The listing builds one solid part. Answer for the finished solid, in the listing's coordinates (mm). Face numbers are marked on the shaded views. A direction names the side the tool comes from. Round coordinates to 2 decimals unless told otherwise and drop trailing zeros. Order: outer loops, then holes, each group sorted by start corner. A loop starts at its lowest first (then second) coordinate and runs counter-clockwise, first axis right, second up. Notation, with made-up numbers: (-21, 56.25) -> (1, 56.25) arc R9 ccw to (1, 73.25) -> close; hole circle Ø2 at (28, 35.5). An arc over 180 degrees is marked (long way). Return JSON: item names as keys, results as strings. Group by question number.
(1) Each of these flat-tipped pins is pushed along its axis until it touches: pin 1 (1 mm diameter, centred on x = 22.5, y = 32, fed in from +Z); pin 2 (6 mm diameter, centred on x = 8, y = 7.5, fed in from -Z); pin 3 (3.5 mm diameter, centred on x = 0, z = 5, fed in from -Y); pin 4 (3 mm diameter, centred on y = 41, z = 48.5, fed in from +X). Where does it stop, or does it pass through?
(2) Determine the mould class of the marked faces 4, 5 and 6 for opening direction Y: +Y half, -Y half, draft (parallel to the pull), parting line (faces both ways), or undercut.
(3) Consider line 1 (X direction, y = -7.5, z = 28); line 2 (Z direction, x = 0, y = 8.35); line 3 (Z direction, x = 0, y = -8.7). Determine where each line is inside the solid, lowest interval first. Write a range as [from, to].
(4) Which of the six approach directions +Z, -Z, +X, -X, +Y, -Y give full straight-line access (tool end or side, diameter ignored) to the marked faces 1, 2 and 3?
(5) The part is cut by section B-B (x = 0). Determine the outline of the cut face in (y, z), plus the area to 3 significant figures.
(6) The part is cut by section C-C (y = 0). Determine the outline of the cut face in (x, z), plus the area to 3 significant figures.
(7) The part is cut by section D-D (x = 15). Determine the outline of the cut face in (y, z).
Autodesk Inventor part; units mm, degrees
ref_plane "Plan de construction2" through (0, -8.75, 15.1554) normal (0, -0.5, 0.8660254) x (1, 0, 0)
ref_plane "Plan de construction4" through (0, -10, 10) normal (0, -0.7071068, 0.7071068) x (1, 0, 0)
ref_plane "Plan de construction7" through (0, 10, 30) normal (0, -0.5, 0.8660254) x (1, 0, 0)
sketch "Esquisse1" plane through (0, 0, 0) normal (0, 0, 1) x (1, 0, 0)
  circle A0 centre (0, 0) radius 8
  circle A1 centre (0, 0) radius 9
  dimension "d0" = 16
  dimension "d1" = 18
extrude "Extrusion1" add sketch "Esquisse1" along normal blind 10
sketch "Esquisse2" plane through (0, 0, 0) normal (1, 0, 0) x (0, 1, 0)
  line L0 (9, 10) -> (-9, 10)
  line L1 (0, 10) -> (0, 25)
  line L2 (9, 10) -> (-9, 10)
  line L3 (0, 10) -> (10, 10)
  line L4 (10, 10) -> (10, 30)
  line L5 (10, 30) -> (-10, 30)
  line L6 (-10, 30) -> (-10, 10)
  line L7 (-10, 10) -> (0, 10)
  point P0 (0, 0)
  dimension "d26" = 10
  dimension "d27" = 20
  dimension "d28" = 20
  dimension "d29" = 90
extrude "Extrusion2" add sketch "Esquisse2" along normal mid plane 20
fillet "Congé1" radius 2 1 edges at (-9, 0, 10)
sketch "Esquisse4" plane through (0, 0, 0) normal (0, 1, 0) x (-1, 0, 0)
  line L0 (9, 0) -> (-9, 0)
  line L1 (9, 0) -> (0, 0)
  line L2 (0, 0) -> (0, 5)
  line L3 (0, 0) -> (5, 0) construction
  dimension "d14" = 9
  dimension "d15" = 5
  dimension "d16" = 90
hole "Perçage1" at (0, 0, 5) direction (0, -1, 0) diameter 4 end through all both
ref_plane "Plan de construction2" through (0, -8.75, 15.1554) normal (0, -0.5, 0.8660254) x (1, 0, 0)
ref_plane "Plan de construction1" through (0, 0, 0) normal (0, -0.5, 0.8660254) x (1, 0, 0)
ref_plane "Plan de construction4" through (0, -10, 10) normal (0, -0.7071068, 0.7071068) x (1, 0, 0)
ref_plane "Plan de construction3" through (0, 0, 0) normal (0, -0.7071068, 0.7071068) x (1, 0, 0)
sketch "Esquisse6" plane through (0, -10, 10) normal (0, -0.7071068, 0.7071068) x (1, 0, 0)
  line L0 (-10, 28.2843) -> (-10, 14.1421)
  line L1 (10, 14.1421) -> (10, 0)
  line L2 (-10, 28.2843) -> (10, 28.2843)
  line L3 (10, 28.2843) -> (10, 0)
  line L4 (10, 0) -> (-10, 0)
  line L5 (-10, 0) -> (-10, 28.2843)
  line L6 (-10, 28.2843) -> (10, 28.2843)
  line L7 (10, 14.1421) -> (10, 28.2843)
  line L8 (4.5826, 14.1421) -> (10, 14.1421)
  line L9 (-10, 14.1421) -> (-4.5826, 14.1421)
  line L10 (-10, 28.2843) -> (-10, 14.1421)
  point P0 (0, 0)
extrude "Extrusion4" add sketch "Esquisse6" along normal blind 25
fillet "Congé4" radius 20 1 edges at (0, -27.6777, 27.6777)
ref_plane "Plan de construction5" through (0, 10, 30) normal (0, 0.8660254, 0.5) x (1, 0, 0)
ref_plane "Plan de construction7" through (0, 10, 30) normal (0, -0.5, 0.8660254) x (1, 0, 0)
ref_plane "Plan de construction6" through (0, 1.3397, 25) normal (0, 0.8660254, 0.5) x (1, 0, 0)
sketch "Esquisse18" plane through (0, 1.3397, 25) normal (0, 0.8660254, 0.5) x (1, 0, 0)
  line L0 (10, -0.0001) -> (-10, -0.0001)
  line L1 (-10, -0.0001) -> (-10, -24.1482)
  line L2 (10, -24.1482) -> (-10, -24.1482)
  line L3 (10, -0.0001) -> (10, -24.1482)
  line L4 (10, -0.0001) -> (-10, -0.0001)
  line L5 (-10, -0.0001) -> (-10, -24.1482)
  line L6 (10, -24.1482) -> (-10, -24.1482)
  line L7 (10, -0.0001) -> (10, -24.1482)
  point P0 (0, 20.9808)
extrude "Extrusion14" add sketch "Esquisse18" along normal blind 60
fillet "Congé6" radius 5 1 edges at (0, -10.7344, 45.913)
sketch "Esquisse19" plane through (10, 0, 0) normal (1, 0, 0) x (0, 0, -1)
  line L0 (-30, 10) -> (-55.0001, 53.3012)
  line L1 (-55.0001, 53.3012) -> (-65.4564, 47.2642)
  line L2 (-47.3761, -8.2002) -> (-75.913, 41.2272)
  line L3 (-65.4564, 47.2642) -> (-58.4714, 35.1659)
  circle A0 centre (-58.4714, 35.1659) radius 4.1
  point P0 (0, 0)
  dimension "d76" = 12.074
  dimension "d77" = 13.97
  dimension "d78" = 8.2
extrude "Extrusion15" add sketch "Esquisse19" along normal blind 20
sketch "Esquisse20" plane through (10, 0, 0) normal (1, 0, 0) x (0, 0, -1)
  circle A0 centre (-58.4714, 35.1659) radius 4.1
  circle A1 centre (-58.4714, 35.1659) radius 4.75
  point P0 (0, 0)
  dimension "d81" = 9.5
extrude "Extrusion16" add sketch "Esquisse20" along normal blind 2
fillet "Congé7" radius 5 2 edges at (0, 53.3012, 55.0001) (0, 41.2272, 75.913)
properties part number "bielle roue milieu autre côté"
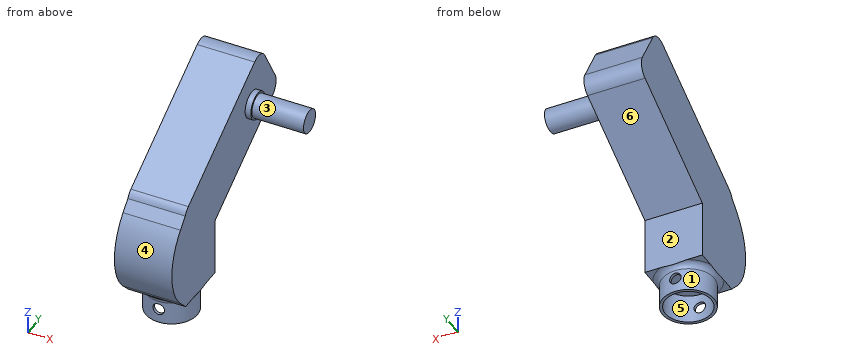
Answer below:
{
 "1": {"pin 1": "stops at z = 61.59", "pin 2": "stops at z = 0", "pin 3": "passes through", "pin 4": "stops at x = 10"},
 "2": {"face 4": "-Y half", "face 5": "undercut", "face 6": "+Y half"},
 "3": {"line 1": "x = [-10, 10]", "line 2": "z = [0, 3], [7, 56.93]", "line 3": "z = [0, 3], [7, 47.05]"},
 "4": {"face 1": "-Z", "face 2": "-Z, +X, -X, +Y", "face 3": "+X"},
 "5": {"outline": "(-13.54, 13.54) -> (-10, 10) -> (-10, 9.73) arc R2 cw to (-9, 8) -> (-9, 7) -> (-8, 7) -> (-8, 10) -> (8, 10) -> (8, 7) -> (9, 7) -> (9, 8) arc R2 cw to (10, 9.73) -> (10, 30) -> (48.97, 52.5) arc R5 ccw to (50.8, 59.33) -> (43.73, 71.58) arc R5 ccw to (36.9, 73.41) -> (-8.2, 47.38) arc R5 ccw to (-10.26, 45.09) -> (-13.54, 41.82) arc R20 ccw to start; (-9, 0) -> (-8, 0) -> (-8, 3) -> (-9, 3) -> close; (8, 0) -> (9, 0) -> (9, 3) -> (8, 3) -> close", "area": "2,110 mm²"},
 "6": {"outline": "(-10, 9.73) arc R2 cw to (-9, 8) -> (-9, 0) -> (-8, 0) -> (-8, 10) -> (8, 10) -> (8, 0) -> (9, 0) -> (9, 8) arc R2 cw to (10, 9.73) -> (10, 52.11) -> (-10, 52.11) -> close", "area": "864 mm²"},
 "7": {"outline": "circle Ø8.2 at (35.17, 58.47)"}
}
